Build history of the part. All positions in model axes, mm. Round coordinates to 2 decimals unless told otherwise and drop trailing zeros. Loops run counter-clockwise (first coordinate to the right, second up) from the corner with the lowest first, then second, coordinate; pieces in that order, holes last. Notation, with made-up numbers: (65.5, -8.5) - (110.5, -8.5) arc R10 ccw to (110.5, 6.5) - close; hole circle Ø7 at (19, 88). An arc over 180 degrees is marked (long way). Use one line per item in the form item = value. Start each with the question number.
Q1. Pin check, flat tips, straight feed: pin 1 (3 mm diameter, centred on x = 7, z = -7, fed in from -Y); pin 2 (2 mm diameter, centred on y = -57, z = -0.5, fed in from -X); pin 3 (1 mm diameter, centred on x = -2, y = 107.5, fed in from +Z). Stop position of each tip, or through.
Q2. Saw through at A-A (y = 177.5). Give the cut face in (x, z), then the cut area to 3 significant figures.
Q3. Drill centre lines: line 1 (X direction, y = -57, z = -7); line 2 (Z direction, x = -7, y = -74); line 3 (X direction, y = 20.5, z = -3.5). Where is each one in solid material? Low to high.
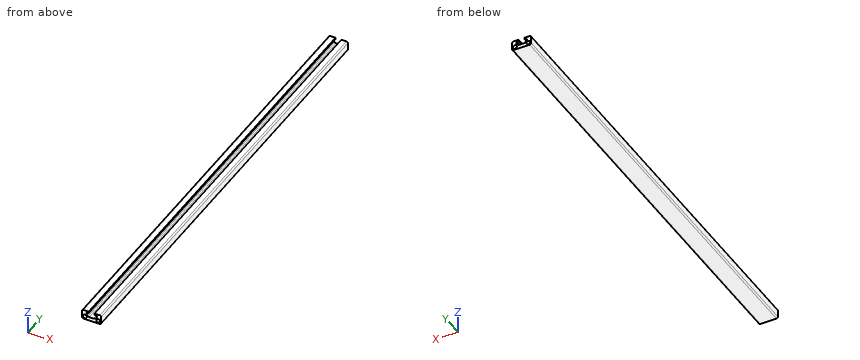
```python
from build123d import *

# Parameters (mm, degrees)
SKETCH1_R           = 2
BOSS_EXTRUDE1_DEPTH = 477


with BuildPart() as part:
    # Sketch1 → Boss-Extrude1 (new body)
    with BuildSketch(Plane(origin=(0, 238.5, 0), x_dir=(1, 0, 0), z_dir=(0, 1, 0))):
        with BuildLine():
            Line((-3.1, 1.8), (-4.95, 1.8))
            ThreePointArc((-4.95, 1.8), (-5.303553391, 1.946446609), (-5.45, 2.3))
            Line((-5.45, 2.3), (-5.45, 3.692893219))
            ThreePointArc((-5.45, 3.692893219), (-5.411939766, 3.884234935), (-5.303553391, 4.046446609))
            Line((-5.303553391, 4.046446609), (-3.835786438, 5.514213562))
            ThreePointArc((-3.835786438, 5.514213562), (-3.18693974, 5.947759065), (-2.421572875, 6.1))
            Line((-2.421572875, 6.1), (2.421572875, 6.1))
            ThreePointArc((2.421572875, 6.1), (3.18693974, 5.947759065), (3.835786438, 5.514213562))
            Line((3.835786438, 5.514213562), (5.303553391, 4.046446609))
            ThreePointArc((5.303553391, 4.046446609), (5.411939766, 3.884234935), (5.45, 3.692893219))
            Line((5.45, 3.692893219), (5.45, 2.3))
            ThreePointArc((5.45, 2.3), (5.303553391, 1.946446609), (4.95, 1.8))
            Line((4.95, 1.8), (3.1, 1.8))
            Line((3.1, 1.8), (3.1, 0))
            Line((3.1, 0), (8.5, 0))
            ThreePointArc((8.5, 0), (9.560660172, 0.439339828), (10, 1.5))
            Line((10, 1.5), (10, 8.5))
            ThreePointArc((10, 8.5), (9.560660172, 9.560660172), (8.5, 10))
            Line((8.5, 10), (-8.5, 10))
            ThreePointArc((-8.5, 10), (-9.560660172, 9.560660172), (-10, 8.5))
            Line((-10, 8.5), (-10, 1.5))
            ThreePointArc((-10, 1.5), (-9.560660172, 0.439339828), (-8.5, 0))
            Line((-8.5, 0), (-3.1, 0))
            Line((-3.1, 0), (-3.1, 1.8))
        make_face()
        with Locations((-7, 7)):
            Circle(SKETCH1_R, mode=Mode.SUBTRACT)
        with Locations((7, 7)):
            Circle(SKETCH1_R, mode=Mode.SUBTRACT)
    extrude(amount=-BOSS_EXTRUDE1_DEPTH)


solid = part.part
```
Report:
q1.pin_1 = through
q1.pin_2 = -10
q1.pin_3 = -6.1
q2.outline = (-10, -8.5) arc R1.5 ccw to (-8.5, -10) - (8.5, -10) arc R1.5 ccw to (10, -8.5) - (10, -1.5) arc R1.5 ccw to (8.5, 0) - (3.1, 0) - (3.1, -1.8) - (4.95, -1.8) arc R0.5 cw to (5.45, -2.3) - (5.45, -3.69) arc R0.5 cw to (5.3, -4.05) - (3.84, -5.51) arc R2 cw to (2.42, -6.1) - (-2.42, -6.1) arc R2 cw to (-3.84, -5.51) - (-5.3, -4.05) arc R0.5 cw to (-5.45, -3.69) - (-5.45, -2.3) arc R0.5 cw to (-4.95, -1.8) - (-3.1, -1.8) - (-3.1, 0) - (-8.5, 0) arc R1.5 ccw to (-10, -1.5) - close; hole circle Ø4 at (-7, -7); hole circle Ø4 at (7, -7)
q2.area = 120 mm²
q3.line_1 = -10 to -9, -5 to 5, 9 to 10
q3.line_2 = -10 to -9, -5 to 0
q3.line_3 = -10 to -5.45, 5.45 to 10
